from build123d import *

# Parameters (mm, degrees)
F0_W     = 50
F0_H     = 34
F1_DEPTH = 5
F2_W     = 46
F2_H     = 30
F3_DEPTH = 3
F5_DEPTH = 2


with BuildPart() as f1:
    # F0 (on Top) → F1 (new body)
    with BuildSketch(Plane.XY):
        Rectangle(F0_W, F0_H)
    extrude(amount=F1_DEPTH)

    # F2 (on face) → F3 (cut)
    with BuildSketch(Plane.XY.offset(5)):
        Rectangle(F2_W, F2_H)
    extrude(amount=-F3_DEPTH, mode=Mode.SUBTRACT)

    # F4 (on face) → F5 (cut)
    with BuildSketch(Plane.XY.offset(2)):
        Polygon((-9, 12), (-21, 12), (-21, 9), (-15, 9), (-15, 6), (-9, 6), align=None)
        Polygon((21, 12), (9, 12), (9, 9), (15, 9), (15, 6), (21, 6), align=None)
        Polygon((-15, -9), (-21, -9), (-21, -12), (-9, -12), (-9, -6), (-15, -6), align=None)
        Polygon((15, -9), (9, -9), (9, -12), (21, -12), (21, -6), (15, -6), align=None)
    extrude(amount=-F5_DEPTH, mode=Mode.SUBTRACT)


solid = f1.part
Geometry: final body of the model. Coordinates: model frame, mm. A direction names the side the tool comes from. Round coordinates to 2 decimals unless told otherwise and drop trailing zeros. Loops run counter-clockwise (first coordinate to the right, second up) from the corner with the lowest first, then second, coordinate; pieces in that order, holes last. Notation, with made-up numbers: M 76.5,-5 L 109.5,-5 A20 ccw 109.5,29 Z; hole C 21.5,19.5 d4. An arc over 180 degrees is marked long. Put each result on its own line as item: value. Start each with the question number.
(1) Contact query for flat-ended pins moving along their axis: pin 1 Ø4 at (x, y) = (7.5, -1) entering from +Z; pin 2 Ø8 at (x, y) = (-3, 6.5) entering from -Z. Output: stop coordinate, or through.
(2) Set-up query: faces 5 (the face through (-9, 9, 1)), 6 (the face through (0, 15, 4)). Return all of +Z, -Z, +X, -X, +Y, -Y with unobstructed straight access to the full face (end or side cutting, diameter ignored); none if empty.
(3) Section query A-A (x = -12). Return loops of the section in (y, z).
(4) Material intervals for line 1 along Y through (x, z) = (12.5, 1.85); line 2 along Y through (x, z) = (-13, 1.2); line 3 along Y through (x, z) = (-8, 3.65), sorted ascending. Write a range as [from, to].
(5) Section query B-B (y = 11). Return loops of the section in (x, z), then the cut area to 3 significant figures.
(6) Section query D-D (z = 1.4). Return loops of the section in (x, y), then the cut area to 3 significant figures.
(7) Draft query along X for faces 1 (the face through (0, 17, 2)), 2 (the face through (12, 9, 1)), 3 (the face through (9, 11, 1)), 4 (the face through (25, 0, 2)). Return one class per face: +X half, -X half, draft (parallel to the pull), parting line (faces both ways), or undercut.
(8) Section query C-C (z = 4.3). Return loops of the section in (x, y), then the cut area to 3 significant figures.
Findings below:
1. pin 1: stops at z = 2
1. pin 2: stops at z = 0
2. face 5: +Z, -Z
2. face 6: +Z
3. outline: M -17,0 L -12,0 L -12,2 L -15,2 L -15,5 L -17,5 Z; M -6,0 L 6,0 L 6,2 L -6,2 Z; M 12,0 L 17,0 L 17,5 L 15,5 L 15,2 L 12,2 Z
4. line 1: y = [-17, -12], [-9, 9], [12, 17]
4. line 2: y = [-17, -12], [-6, 6], [12, 17]
4. line 3: y = [-17, -15], [15, 17]
5. outline: M -25,0 L -21,0 L -21,2 L -23,2 L -23,5 L -25,5 Z; M -9,0 L 9,0 L 9,2 L -9,2 Z; M 21,0 L 25,0 L 25,5 L 23,5 L 23,2 L 21,2 Z
5. area: 64.0 mm2
6. outline: M -25,-17 L 25,-17 L 25,17 L -25,17 Z; hole M -21,-12 L -9,-12 L -9,-6 L -15,-6 L -15,-9 L -21,-9 Z; hole M -21,9 L -15,9 L -15,6 L -9,6 L -9,12 L -21,12 Z; hole M 9,-12 L 21,-12 L 21,-6 L 15,-6 L 15,-9 L 9,-9 Z; hole M 9,9 L 15,9 L 15,6 L 21,6 L 21,12 L 9,12 Z
6. area: 1,480 mm2
7. face 1: draft
7. face 2: undercut
7. face 3: undercut
7. face 4: +X half
8. outline: M -25,-17 L 25,-17 L 25,17 L -25,17 Z; hole M -23,-15 L 23,-15 L 23,15 L -23,15 Z
8. area: 320 mm2
